Could you check a few things on this model? Use its own coordinates, in mm. A direction names the side the tool comes from. Round coordinates to 2 decimals unless told otherwise and drop trailing zeros. Loops run counter-clockwise (first coordinate to the right, second up) from the corner with the lowest first, then second, coordinate; pieces in that order, holes last. Notation, with made-up numbers: M 31.5,65 L 72.5,65 A18 ccw 72.5,93 Z; hole C -8.5,-0.5 d1. An arc over 180 degrees is marked long. Answer in a Markdown table with one row per item.
```python
from build123d import *

# Parameters (mm, degrees)
CUT_EXTRUDE_1_DEPTH = 10
SKETCH_3_R          = 4.5
CUT_EXTRUDE_2_DEPTH = 2
CHAMFER_1_SIZE      = 0.5


with BuildPart() as part:
    # Эскиз1 → Повернуть1 (revolve)
    with BuildSketch(Plane.XY, mode=Mode.PRIVATE) as revolve_1_sk:
        Polygon((0, 0), (-6, 0), (-6, -2.952380952), (-4.952380952, -4), (-3.5, -4), (-3.5, -5.483974596), (-3, -6.35), (-0.5, -6.35), (0, -5.483974596), align=None)
    revolve(revolve_1_sk.sketch.rotate(Axis((0, 0, 0), (-1, 0, 0)), 180), axis=Axis((0, 0, 0), (-1, 0, 0)))

    # Эскиз2 → Вырез-Вытянуть1 (cut)
    with BuildSketch(Plane(origin=(0, 0, 0), x_dir=(0, 0, -1), z_dir=(1, 0, 0))):
        with BuildLine():
            Line((-5.499261314, 3.175), (0, 6.35))
            ThreePointArc((0, 6.35), (-3.175, 5.499261314), (-5.499261314, 3.175))
        make_face()
        with BuildLine():
            ThreePointArc((5.499261314, 3.175), (3.175, 5.499261314), (0, 6.35))
            Line((0, 6.35), (5.499261314, 3.175))
        make_face()
        with BuildLine():
            ThreePointArc((6.35, 0), (6.133628997, 1.643500936), (5.499261314, 3.175))
            Line((5.499261314, 3.175), (5.499261314, -3.175))
            ThreePointArc((5.499261314, -3.175), (6.133628997, -1.643500936), (6.35, 0))
        make_face()
        with BuildLine():
            ThreePointArc((0, -6.35), (3.175, -5.499261314), (5.499261314, -3.175))
            Line((5.499261314, -3.175), (0, -6.35))
        make_face()
        with BuildLine():
            Line((0, -6.35), (-5.499261314, -3.175))
            ThreePointArc((-5.499261314, -3.175), (-3.175, -5.499261314), (0, -6.35))
        make_face()
        with BuildLine():
            Line((-5.499261314, -3.175), (-5.499261314, 3.175))
            ThreePointArc((-5.499261314, 3.175), (-6.35, 0), (-5.499261314, -3.175))
        make_face()
    extrude(amount=-CUT_EXTRUDE_1_DEPTH, mode=Mode.SUBTRACT)

    # Эскиз3 → Вырез-Вытянуть2 (cut)
    with BuildSketch(Plane(origin=(0, 0, 0), x_dir=(0, 0, -1), z_dir=(1, 0, 0))):
        with Locations(Location((0, 0, 0), (0, 0, 90))):
            Circle(SKETCH_3_R)
    extrude(amount=-CUT_EXTRUDE_2_DEPTH, mode=Mode.SUBTRACT)

    # Фаска1
    chamfer_1_edges = [part.edges().sort_by_distance(p)[0] for p in [
        (0, -4.5, 0),
    ]]
    chamfer(chamfer_1_edges, length=CHAMFER_1_SIZE)


solid = part.part
```
1) I need wall thicknesses on line 1 (Z direction, x = -1.5, y = 0); line 2 (X direction, y = -3.5, z = -2.5); line 3 (Z direction, x = -1.75, y = -2.5). Which ranges of each line are inside material? Lowest first, please.
Computed:
| item | result |
|---|---|
| line 1 | z = -5.5 to -4.5, 4.5 to 5.5 |
| line 2 | x = -3.5 to -2 |
| line 3 | z = -5.5 to -3.74, 3.74 to 5.5 |
2) I want a section at C-C, the plane x = -4.15. Please give me the cut outline in (y, z).
Computed:
| item | result |
|---|---|
| outline | C 0,0 d8 |
3) Will this pin go through, and if not, where does the flat tip stop? P1, Ø1, axis at y = -1, z = -3.5, coming from the +X side.
Computed:
| item | result |
|---|---|
| P1 | stops at x = -2 |
4) I want a section at A-A, the plane x = -1.5. Please give me the cut outline in (y, z) (3 decimals).
Computed:
| item | result |
|---|---|
| outline | M -6.35,0 L -3.175,-5.499 L 3.175,-5.499 L 6.35,0 L 3.175,5.499 L -3.175,5.499 Z; hole C 0,0 d9 |
5) Which directions (+Z, -Z, +X, -X, +Y, -Y) give clear straight access to the entire face, cutting with the end or side of a thin tool? Please do faces 1 (the face through (-2, 0, 0)), 2 (the face through (-6, 0, 0)), 3 (the face through (-3.5, 4, 2)).
Computed:
| item | result |
|---|---|
| face 1 | +X |
| face 2 | +Z, -Z, -X, +Y, -Y |
| face 3 | -X |
